Input: part model. Units: mm. Frame: model coordinates. A direction names the side the tool comes from. Give positions to 0.01 mm unless a question says otherwise; leave off trailing zeros. Loops run counter-clockwise (first coordinate to the right, second up) from the corner with the lowest first, then second, coordinate; pieces in that order, holes last. Notation, with made-up numbers: (26, 14.25) - (49, 14.25) arc R10 ccw to (49, 18.25) - close; hole circle Ø3 at (-25.75, 74.5). An arc over 180 degrees is marked (long way). Answer as a JSON object with one key per item and string values.
from build123d import *
from OCP.BRepFilletAPI import BRepFilletAPI_MakeChamfer

# Parameters (mm, degrees)
EXTRUDE_1_DEPTH     = 19
CUT_EXTRUDE_1_REACH = 28.26
SKETCH_6_W          = 20
SKETCH_6_H          = 6
CHAMFER_1_SIZE      = 1.4
CHAMFER_1_SIZE2     = 0.808290377
CUT_EXTRUDE_3_REACH = 28.26
SKETCH_9_W          = 10
SKETCH_9_H          = 3.85
FILLET_4_R          = 1
EXTRUDE_4_DEPTH     = 3.5
SKETCH_11_R         = 10
CUT_EXTRUDE_4_DEPTH = 1.5
CHAMFER_2_SIZE      = 6
CHAMFER_2_SIZE_2    = 2.183821406
SHELL_START         = -1.98
SHELL_4_DEPTH       = 3.96
SHELL_START_2       = 0.02
SHELL_4_2_DEPTH     = 12.394886134
SHELL_START_3       = 12.360630137
SHELL_4_3_DEPTH     = 1.52
SKETCH_12_R         = 0.95
CUT_EXTRUDE_5_DEPTH = 42.164304926


with BuildPart() as part:
    # 草圖1 → 填料-伸長1 (new, symmetric)
    with BuildSketch(Plane(origin=(0, 0, 0), x_dir=(0, 0, -1), z_dir=(1, 0, 0))):
        Polygon((0, 12.8), (0, 0), (7.9, 0), (7.9, 1.5), (9.4, 1.5), (9.4, -1.5), (-1.5, -1.5), (-1.5, 14), (3.85, 14), (3.85, 12), (2.65, 12), (2.65, 12.8), align=None)
    extrude(amount=EXTRUDE_1_DEPTH, both=True)

    # 草圖6 → 除料-伸長1 (cut, up to next)
    with BuildSketch(Plane(origin=(0, -1.5, 0), x_dir=(1, 0, 0), z_dir=(0, 1, 0)), mode=Mode.PRIVATE) as cut_extrude_1_sk1:
        with Locations((0, 6.4)):
            Rectangle(SKETCH_6_W, SKETCH_6_H)
    cut_extrude_1_tool1 = extrude(cut_extrude_1_sk1.sketch, amount=CUT_EXTRUDE_1_REACH, mode=Mode.PRIVATE) & part.part
    add(cut_extrude_1_tool1.solids().sort_by_distance((0, -1.5, -6.4))[0], mode=Mode.SUBTRACT)

    # 導角1: one chamfer whose edges measure the first distance from different faces: ONE call of the kernel's chamfer builder (chamfer() names one face for all edges)
    chamfer_1_edges_1 = [part.edges().sort_by_distance(p)[0] for p in [
        (14.5, 1.5, -9.4),
    ]]
    chamfer_1_side_1 = [part.faces().sort_by_distance(p)[0] for p in [
        (14.5, 1.5, -8.65),
    ]]
    chamfer_1_edges_2 = [part.edges().sort_by_distance(p)[0] for p in [
        (-14.5, 1.5, -9.4),
    ]]
    chamfer_1_side_2 = [part.faces().sort_by_distance(p)[0] for p in [
        (-14.5, 1.5, -8.65),
    ]]
    chamfer_1 = BRepFilletAPI_MakeChamfer(part.part.solid().wrapped)
    for e in chamfer_1_edges_1:
        chamfer_1.Add(CHAMFER_1_SIZE, CHAMFER_1_SIZE2, e.wrapped, chamfer_1_side_1[0].wrapped)  # the first distance lies on this face
    for e in chamfer_1_edges_2:
        chamfer_1.Add(CHAMFER_1_SIZE, CHAMFER_1_SIZE2, e.wrapped, chamfer_1_side_2[0].wrapped)  # the first distance lies on this face
    add(Compound.cast(chamfer_1.Shape()), mode=Mode.REPLACE)

    # 草圖9 → 除料-伸長3 (cut, up to next)
    with BuildSketch(Plane(origin=(0, 14, 0), x_dir=(1, 0, 0), z_dir=(0, 1, 0)), mode=Mode.PRIVATE) as cut_extrude_3_sk1:
        with Locations((0, 1.925)):
            Rectangle(SKETCH_9_W, SKETCH_9_H)
    cut_extrude_3_tool1 = extrude(cut_extrude_3_sk1.sketch, amount=-CUT_EXTRUDE_3_REACH, mode=Mode.PRIVATE) & part.part
    add(cut_extrude_3_tool1.solids().sort_by_distance((0, 14, -1.925))[0], mode=Mode.SUBTRACT)

    # 圓角4
    fillet_4_edges = [part.edges().sort_by_distance(p)[0] for p in [
        (14.5, 0.691709623, -9.4),
        (-14.5, 0.691709623, -9.4),
    ]]
    fillet(fillet_4_edges, radius=FILLET_4_R)

    # 草圖10 → 填料-伸長4 (add, symmetric)
    with BuildSketch(Plane(origin=(0, 0, 0), x_dir=(0, 0, -1), z_dir=(1, 0, 0))):
        with BuildLine():
            Line((-1.5, -1.5), (-27.5, -1.5))
            ThreePointArc((-27.5, -1.5), (-31.462172303, 1.951191618), (-28.587236685, 6.34940468))
            Line((-28.587236685, 6.34940468), (-1.5, 14))
            Line((-1.5, 14), (-1.5, -1.5))
        make_face()
    extrude(amount=EXTRUDE_4_DEPTH, both=True)

    # 草圖11 → 除料-伸長4 (cut, symmetric)
    with BuildSketch(Plane(origin=(0, 0, 0), x_dir=(0, 0, -1), z_dir=(1, 0, 0))):
        with Locations((-27.5, 2.5)):
            Circle(SKETCH_11_R)
    extrude(amount=CUT_EXTRUDE_4_DEPTH, both=True, mode=Mode.SUBTRACT)

    # 導角2
    # the kernel refuses this chamfer: 6, 2.183821406 mm, written as the material it adds along each edge
    with BuildSketch(Plane(origin=(-3.5, 14, 1.5), x_dir=(0, 0, 1), z_dir=(0, -1, 0))) as chamfer_2_piece_1_section:
        Polygon((CHAMFER_2_SIZE, 0), (0, CHAMFER_2_SIZE_2), (0, 0), align=None)
    chamfer_2_piece_1 = extrude(amount=15.5, mode=Mode.PRIVATE)
    chamfer_2_piece_1 = split(chamfer_2_piece_1, bisect_by=Plane(origin=(-3.5, 14, 1.5), z_dir=(0, -0.9623511699869516, -0.2718091713403826)), keep=Keep.TOP, mode=Mode.PRIVATE)
    add(chamfer_2_piece_1)
    with BuildSketch(Plane(origin=(3.5, 14, 1.5), x_dir=(0, 0, 1), z_dir=(0, -1, 0))) as chamfer_2_piece_2_section:
        Polygon((CHAMFER_2_SIZE, 0), (0, -CHAMFER_2_SIZE_2), (0, 0), align=None)
    chamfer_2_piece_2 = extrude(amount=15.5, mode=Mode.PRIVATE)
    chamfer_2_piece_2 = split(chamfer_2_piece_2, bisect_by=Plane(origin=(3.5, 14, 1.5), z_dir=(0, -0.9623511699869516, -0.2718091713403826)), keep=Keep.TOP, mode=Mode.PRIVATE)
    add(chamfer_2_piece_2)

    # 薄殼4: read off the stored shape, not the designer's step
    # 薄殼4 outline → 薄殼4 (cut)
    with BuildSketch(Plane.YZ.offset(SHELL_START)):
        with BuildLine():
            Line((0.02, 1.52), (12.414886134, 1.52))
            Line((12.414886134, 1.52), (7.944453878, 17.347743011))
            ThreePointArc((7.944453878, 17.347743011), (4.08056814, 16.088943767), (0.02, 16.250111112))
            Line((0.02, 16.250111112), (0.02, 1.52))
        make_face()
    extrude(amount=SHELL_4_DEPTH, mode=Mode.SUBTRACT)

    # Shell 4 2 outline → Shell 4 2 (cut)
    with BuildSketch(Plane(origin=(0, 0, 0), x_dir=(1, 0, 0), z_dir=(0, 1, 0)).offset(SHELL_START_2)):
        Polygon((4.058991787, -1.52), (1.98, -1.52), (1.98, -7.231982989), align=None)
        Polygon((-1.98, -1.52), (-4.058991787, -1.52), (-1.98, -7.231982989), align=None)
    extrude(amount=SHELL_4_2_DEPTH, mode=Mode.SUBTRACT)

    # Shell 4 3 outline → Shell 4 3 (add)
    with BuildSketch(Plane(origin=(0, 0, 0), x_dir=(1, 0, 0), z_dir=(0, 0.9623511699869516, 0.2718091713403829)).offset(SHELL_START_3)):
        Polygon((4.058991787, 1.911706134), (-4.058991787, 1.911706134), (-1.98, -4.023739437), (-1.98, -14.535245358), (1.98, -14.535245358), (1.98, -4.023739437), align=None)
    extrude(amount=SHELL_4_3_DEPTH)

    # 草圖12 → 除料-伸長5 (cut, through all)
    with BuildSketch(Plane(origin=(3.5, 0, 0), x_dir=(0, 0, -1), z_dir=(1, 0, 0))):
        with Locations((-27.5, 2.5)):
            Circle(SKETCH_12_R)
    extrude(amount=-CUT_EXTRUDE_5_DEPTH, mode=Mode.SUBTRACT)


solid = part.part
Item 1: Material intervals for line 1 (X direction, y = 7.75, z = 15); line 2 (X direction, y = 7.5, z = 20.5); line 3 (Y direction, x = -14, z = -2), sorted ascending. Write a range as [from, to].
Geometry check:
{"line 1": "x = [-3.5, -1.98], [1.98, 3.5]", "line 2": "x = [-3.5, -1.5], [1.5, 3.5]", "line 3": "y = [-1.5, 0], [12.8, 14]"}
Item 2: Cut plane A-A (y = 2.5). Return loops of the section in (x, z).
Geometry check:
{"outline": "(-19, 0) - (19, 0) - (19, 1.5) - (5.68, 1.5) - (3.5, 7.5) - (3.5, 26.55) - (1.5, 26.55) - (1.5, 17.5) - (-1.5, 17.5) - (-1.5, 26.55) - (-3.5, 26.55) - (-3.5, 7.5) - (-5.68, 1.5) - (-19, 1.5) - close; (-3.5, 28.45) - (-1.5, 28.45) - (-1.5, 31.5) - (-3.5, 31.5) - close; (1.5, 28.45) - (3.5, 28.45) - (3.5, 31.5) - (1.5, 31.5) - close; hole (-4.06, 1.52) - (4.06, 1.52) - (1.98, 7.23) - (1.98, 15.98) - (-1.98, 15.98) - (-1.98, 7.23) - close"}
Item 3: Contact query for flat-ended pins moving along their axis: P1, Ø1.6, axis at x = 10, y = 13, coming from the -Z side; P2, Ø5, axis at y = 8, z = 13, coming from the +X side; P3, Ø3, axis at y = 1, z = 10.5, coming from the -X side. Output: stop coordinate, or through.
Geometry check:
{"P1": "stops at z = -3.85", "P2": "stops at x = 3.5", "P3": "stops at x = -3.5"}
Item 4: Cut plane B-B (z = -5.5). Return loops of the section in (x, y), then the cut area to 3 significant figures.
Geometry check:
{"outline": "(-19, -1.5) - (-10, -1.5) - (-10, 0) - (-19, 0) - close; (10, -1.5) - (19, -1.5) - (19, 0) - (10, 0) - close", "area": "27.0 mm2"}
Item 5: Access query for faces 5 (the face through (0, 0, -3)), 6 (the face through (15, -1, -9.4)), 7 (the face through (4.577, 6.358, 4.542)), 8 (the face through (-14, 1, -7.9)), 9 (the face through (1.98, 5, 11)). Directions: +Z, -Z, +X, -X, +Y, -Y. A direction counts if a zero-diameter tool reaches every point of the face in a straight line with its end or side. Return the directions, or none.
Geometry check:
{"face 5": "+X, -X", "face 6": "-Z, +X, -X, +Y, -Y", "face 7": "+Z, +X, +Y, -Y", "face 8": "+X, -X, +Y", "face 9": "none"}
Item 6: Cut plane D-D (z = 10.5). Return loops of the section in (x, y).
Geometry check:
{"outline": "(-3.5, -1.5) - (3.5, -1.5) - (3.5, 11.46) - (-3.5, 11.46) - close; hole (-1.98, 0.02) - (1.98, 0.02) - (1.98, 9.88) - (-1.98, 9.88) - close"}
Item 7: Cut plane C-C (x = -10.5). Return loops of the section in (y, z).
Geometry check:
{"outline": "(-1.5, -9.4) - (0.11, -9.4) arc R1 ccw to (0.98, -8.9) - (1.5, -8) - (1.5, -7.9) - (0, -7.9) - (0, 0) - (12.8, 0) - (12.8, -2.65) - (12, -2.65) - (12, -3.85) - (14, -3.85) - (14, 1.5) - (-1.5, 1.5) - close"}
Item 8: Mould query, pull axis X, two halves, no side actions, for faces 1 (the face through (12, 13, -3.85)), 2 (the face through (3.005, 6.131, 4.416)), 3 (the face through (-19, 4.6, 0.5)), 4 (the face through (-1.98, 5, 11)). Classes: released by +X, released by -X, zero draft, split by the parting line, or undercut.
Geometry check:
{"face 1": "zero draft", "face 2": "undercut", "face 3": "released by -X", "face 4": "undercut"}
